Read the model definition and answer for the solid it produces. Units are mm, in the model's axes. Give positions to 0.01 mm unless a question says otherwise; leave off trailing zeros. Loops run counter-clockwise (first coordinate to the right, second up) from the corner with the lowest first, then second, coordinate; pieces in that order, holes last.
(1) Each of these flat-tipped pins is pushed along its axis until it touches: P1, Ø3, axis at x = -33.19, z = -17.32, coming from the +Y side; P2, Ø1, axis at x = -31, y = -2.5, coming from the -Z side. Where does it stop, or does it pass through?
(2) Find section C-C, the plane x = -26. Write down the section's boundary in (y, z) (3 decimals).
(3) Find section B-B, the plane y = -0.75. State how many separate pieces and enclosed holes the cut face has, then the cut area to 3 significant figures.
(4) Find section A-A, the plane x = -57. Write down the section's boundary in (y, z) (3 decimals), then the cut area to 3 significant figures.
(5) Straight lines are drawn through the part: probe 1 along Z at (x, y) = (-42.5, -2.3); probe 2 along Z at (x, y) = (-41.5, -2.2); probe 3 along X at (y, z) = (-2.15, -16). For each, find the intervals that lie inside material, in ascending order.
(6) Find section D-D, the plane x = -52. Write down the section's boundary in (y, z) (3 decimals).
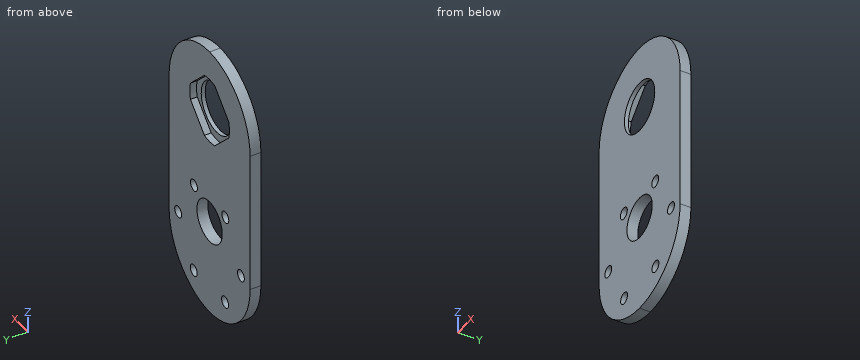
```python
from build123d import *

# Parameters (mm, degrees)
CROQUIS1_W                   = 40
CROQUIS1_H                   = 82
BRIDA_BASE1_DEPTH            = 3.175
CROQUIS6_R                   = 6.25
CORTAR_EXTRUIR17_DEPTH       = 2
CORTAR_EXTRUIR5_START        = -10
CROQUIS5_R                   = 7.5
CROQUIS5_R_2                 = 6.25
CORTAR_EXTRUIR5_DEPTH        = 10
REDONDEO1_R                  = 20
TALADRO_DE_MARGEN_PARA_M31_D = 3.4


# Sheet-metal steps are written as plain solids
with BuildPart() as part:
    # Croquis1 → Brida base1 (new body)
    with BuildSketch(Plane(origin=(0, 0, 0), x_dir=(1, 0, 0), z_dir=(0, 1, 0))):
        with Locations((-40.908481915, 11.276700353)):
            Rectangle(CROQUIS1_W, CROQUIS1_H)
    extrude(amount=-BRIDA_BASE1_DEPTH)

    # Croquis6 → Cortar-Extruir17 (cut)
    with BuildSketch(Plane(origin=(0, 0, 0), x_dir=(1, 0, 0), z_dir=(0, 1, 0))):
        with Locations(Location((-40.908481915, 23.776700353, 0), (0, 0, 270))):
            Circle(CROQUIS6_R)
        with BuildLine():
            Line((-43.469976683, -1.763979135), (-50.367802427, -8.661804879))
            ThreePointArc((-50.367802427, -8.661804879), (-50.708481915, -11.223299647), (-50.367802427, -13.784794415))
            Line((-50.367802427, -13.784794415), (-43.469976683, -20.682620159))
            ThreePointArc((-43.469976683, -20.682620159), (-40.908481915, -21.023299647), (-38.346987147, -20.682620159))
            Line((-38.346987147, -20.682620159), (-31.449161403, -13.784794415))
            ThreePointArc((-31.449161403, -13.784794415), (-31.108481915, -11.223299647), (-31.449161403, -8.661804879))
            Line((-31.449161403, -8.661804879), (-38.346987147, -1.763979135))
            ThreePointArc((-38.346987147, -1.763979135), (-40.908481915, -1.423299647), (-43.469976683, -1.763979135))
        make_face()
    extrude(amount=-CORTAR_EXTRUIR17_DEPTH, mode=Mode.SUBTRACT)

    # Croquis5 → Cortar-Extruir5 (cut)
    with BuildSketch(Plane.XZ.offset(3.175).offset(CORTAR_EXTRUIR5_START)):
        with Locations(Location((-40.908481915, 11.223299647, 0), (0, 0, 270))):
            Circle(CROQUIS5_R)
        with Locations(Location((-40.908481915, -23.776700353, 0), (0, 0, 90))):
            Circle(CROQUIS5_R_2)
    extrude(amount=CORTAR_EXTRUIR5_DEPTH, mode=Mode.SUBTRACT)

    # Redondeo1
    redondeo1_edges = [part.edges().sort_by_distance(p)[0] for p in [
        (-60.908481915, -1.5875, -52.276700353),
        (-20.908481915, -1.5875, -52.276700353),
        (-20.908481915, -1.5875, 29.723299647),
        (-60.908481915, -1.5875, 29.723299647),
    ]]
    fillet(redondeo1_edges, radius=REDONDEO1_R - 0.0001)  # a hair under: the kernel refuses the full size

    # Taladro de margen para M31 (through all)
    with Locations(Plane(origin=(-178.498967671, -3.175, 246.519317109), x_dir=(0.8065687193086877, 0, 0.59114033954108), z_dir=(0, -1, 0))):
        with Locations((-65.46157961, -295.903051669), (-67.078989392, -311.31843313), (-51.302762764, -289.596078899), (-54.537582329, -320.426841821), (-40.378765484, -314.119869051), (-38.761355701, -298.70448759)):
            Hole(TALADRO_DE_MARGEN_PARA_M31_D / 2)


solid = part.part
```
Entries:
1. P1: passes through
1. P2: stops at z = -49.93
2. outline: (-3.175, -45.609) - (0, -45.609) - (0, -32.292) - (-3.175, -32.292) - close; (-3.175, -29.127) - (0, -29.127) - (0, 23.055) - (-3.175, 23.055) - close
3. separate pieces: 1
3. enclosed holes: 8
3. area: 2,490 mm2
4. outline: (-3.175, -44.154) - (0, -44.154) - (0, -32.426) - (-3.175, -32.426) - close; (-3.175, -29.262) - (0, -29.262) - (0, 21.6) - (-3.175, 21.6) - close
4. area: 199 mm2
5. probe 1: z = -52.21 to -29.82, -17.73 to 3.89, 18.55 to 29.66
5. probe 2: z = -52.27 to -30, -17.55 to 3.75, 18.7 to 29.71
5. probe 3: x = -60.91 to -49.67, -47.7 to -34.26, -32.11 to -20.91
6. outline: (-3.175, -48.919) - (0, -48.919) - (0, 26.366) - (-3.175, 26.366) - close
